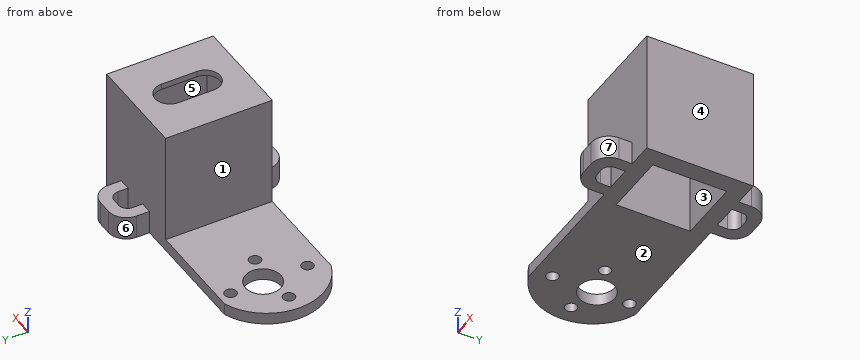
from build123d import *

# Parameters (mm, degrees)
SKETCH2_R            = 1
SKETCH2_R_2          = 3
BOSS_EXTRUDE2_DEPTH  = 2
SKETCH3_W            = 10.8
SKETCH3_H            = 12.5
CUT_EXTRUDE1_DEPTH   = 3
SKETCH4_W            = 17.364181201
SKETCH4_H            = 18
BOSS_EXTRUDE3_DEPTH  = 19
SKETCH5_W            = 10.8
SKETCH5_H            = 12.5
CUT_EXTRUDE2_DEPTH   = 18
BOSS_EXTRUDE4_DEPTH  = 4
FILLET1_R            = 1.5
FILLET2_R            = 3
FILLET1_OF_MIRROR1_R = 1.5
FILLET2_OF_MIRROR1_R = 3
CUT_EXTRUDE3_DEPTH   = 10


with BuildPart() as part:
    # Sketch2 → Boss-Extrude2 (new body)
    with BuildSketch(Plane.XY):
        with BuildLine():
            Line((-18.735484911, 68.428926153), (15.992877491, 68.428926153))
            Line((15.992877491, 68.428926153), (15.992877491, 50.428926153))
            Line((15.992877491, 50.428926153), (-18.735484911, 50.428926153))
            ThreePointArc((-18.735484911, 50.428926153), (-25.000050177, 59.428926153), (-18.735484911, 68.428926153))
        make_face()
        with Locations((-17, 53.428926153)):
            Circle(SKETCH2_R, mode=Mode.SUBTRACT)
        with Locations((-17, 60.928926153)):
            Circle(SKETCH2_R_2, mode=Mode.SUBTRACT)
        with Locations((-22, 59.428926153)):
            Circle(SKETCH2_R, mode=Mode.SUBTRACT)
        with Locations((-17, 66.428926153)):
            Circle(SKETCH2_R, mode=Mode.SUBTRACT)
        with Locations((-12, 59.428926153)):
            Circle(SKETCH2_R, mode=Mode.SUBTRACT)
    extrude(amount=BOSS_EXTRUDE2_DEPTH)

    # Sketch3 → Cut-Extrude1 (cut, through all)
    with BuildSketch(Plane.XY.offset(2)):
        with Locations((7.592877491, 59.428926153)):
            Rectangle(SKETCH3_W, SKETCH3_H)
    extrude(amount=-CUT_EXTRUDE1_DEPTH, mode=Mode.SUBTRACT)

    # Sketch4 → Boss-Extrude3 (add)
    with BuildSketch(Plane.XY.offset(2)):
        with Locations((7.310786891, 59.428926153)):
            Rectangle(SKETCH4_W, SKETCH4_H)
    extrude(amount=BOSS_EXTRUDE3_DEPTH)

    # Sketch5 → Cut-Extrude2 (cut)
    with BuildSketch(Plane(origin=(0, 0, 2), x_dir=(-1, 0, 0), z_dir=(0, 0, -1))):
        with Locations((-7.592877491, 59.428926153)):
            Rectangle(SKETCH5_W, SKETCH5_H)
    extrude(amount=-CUT_EXTRUDE2_DEPTH, mode=Mode.SUBTRACT)

    # Sketch7 → Boss-Extrude4 (add)
    with BuildSketch(Plane(origin=(0, 0, 0), x_dir=(-1, 0, 0), z_dir=(0, 0, -1))):
        Polygon((-11.692877491, 68.428926153), (-9.692877491, 68.428926153), (-9.692877491, 71.628926153), (-5.392877491, 71.628926153), (-5.392877491, 68.428926153), (-3.392877491, 68.428926153), (-3.392877491, 73.628926153), (-11.692877491, 73.628926153), align=None)
    boss_extrude4 = extrude(amount=-BOSS_EXTRUDE4_DEPTH)

    # Fillet1
    fillet1_edges = [part.edges().sort_by_distance(p)[0] for p in [
        (5.392877491, 71.628926153, 2),
        (9.692877491, 71.628926153, 2),
    ]]
    fillet(fillet1_edges, radius=FILLET1_R)

    # Fillet2
    fillet2_edges = [part.edges().sort_by_distance(p)[0] for p in [
        (3.392877491, 73.628926153, 2),
        (11.692877491, 73.628926153, 2),
    ]]
    fillet(fillet2_edges, radius=FILLET2_R)

    # Mirror1: Boss-Extrude4 across plane
    add(boss_extrude4.mirror(Plane.ZX.offset(59.428926153)))

    # Fillet1 of Mirror1
    fillet1_of_mirror1_edges = [part.edges().sort_by_distance(p)[0] for p in [
        (5.392877491, 47.228926153, 2),
        (9.692877491, 47.228926153, 2),
    ]]
    fillet(fillet1_of_mirror1_edges, radius=FILLET1_OF_MIRROR1_R)

    # Fillet2 of Mirror1
    fillet2_of_mirror1_edges = [part.edges().sort_by_distance(p)[0] for p in [
        (3.392877491, 45.228926153, 2),
        (11.692877491, 45.228926153, 2),
    ]]
    fillet(fillet2_of_mirror1_edges, radius=FILLET2_OF_MIRROR1_R)

    # Sketch9 → Cut-Extrude3 (cut)
    with BuildSketch(Plane.XY.offset(21)):
        with BuildLine():
            Line((9.971454774, 62.64486165), (9.971454774, 56.64486165))
            ThreePointArc((9.971454774, 56.64486165), (7.471454774, 54.14486165), (4.971454774, 56.64486165))
            Line((4.971454774, 56.64486165), (4.971454774, 62.64486165))
            ThreePointArc((4.971454774, 62.64486165), (7.471454774, 65.14486165), (9.971454774, 62.64486165))
        make_face()
    extrude(amount=-CUT_EXTRUDE3_DEPTH, mode=Mode.SUBTRACT)


solid = part.part
Input: part model. Units: mm. Frame: model coordinates. Face numbers are marked on the shaded views. A direction names the side the tool comes from. Give positions to 0.01 mm unless a question says otherwise; leave off trailing zeros. Write each loop counter-clockwise with the first axis right and the second up, starting at its lowest first coordinate (ties: lowest second). Pieces come first, ordered by that corner, then holes.
Q1. Section C-C, the plane x = -12. Output: boundary loops of the cut face in (y, z), plus the area to 3 significant figures.
Q2. Pull-direction query (Y, two-part tool) for the marked faces 4, 5, 6 and 7; classes: pulls with the +Y half, pulls with the -Y half, needs draft (parallel to the pull), parting line crosses it, or undercut.
Q3. First-contact query: P1, Ø4, axis at y = 68.5, z = 7.5, coming from the -X side; P2, Ø0.5, axis at y = 69, z = 1.5, coming from the -X side; P3, Ø2.5, axis at y = 49, z = 1.5, coming from the +X side; P4, Ø5, axis at x = -17, y = 60.93, coming from the -Z side. Flat tips, straight axial feed; report the tip coordinate or a pass-through.
Q4. Material intervals for probe 1 along Y at (x, z) = (-17, 0.7); probe 2 along X at (y, z) = (53.75, 16.5); probe 3 along X at (y, z) = (52.75, 19.25), sorted ascending.
Q5. Section A-A, the plane x = -17. Output: boundary loops of the cut face in (y, z), plus the area to 3 significant figures.
Q6. Set-up query: the marked faces 1, 2 and 3. Return all of +Z, -Z, +X, -X, +Y, -Y with unobstructed straight access to the full face (end or side cutting, diameter ignored); none if empty.
Q7. Section B-B, the plane z = 11.75. Output: boundary loops of the cut face in (x, y).
Q8. Section D-D, the plane y = 55. Output: boundary loops of the cut face in (x, z).
Filled in:
1. outline: (50.43, 0) - (58.43, 0) - (58.43, 2) - (50.43, 2) - close; (60.43, 0) - (68.43, 0) - (68.43, 2) - (60.43, 2) - close
1. area: 32.0 mm2
2. face 4: needs draft
2. face 5: undercut
2. face 6: pulls with the +Y half
2. face 7: pulls with the -Y half
3. P1: stops at x = -1.37
3. P2: stops at x = 3.39
3. P3: stops at x = 11.69
3. P4: passes through
4. probe 1: y = 50.43 to 52.43, 54.43 to 57.93, 63.93 to 65.43, 67.43 to 68.43
4. probe 2: x = -1.37 to 2.19, 12.99 to 15.99
4. probe 3: x = -1.37 to 15.99
5. outline: (50.43, 0) - (52.43, 0) - (52.43, 2) - (50.43, 2) - close; (54.43, 0) - (57.93, 0) - (57.93, 2) - (54.43, 2) - close; (63.93, 0) - (65.43, 0) - (65.43, 2) - (63.93, 2) - close; (67.43, 0) - (68.43, 0) - (68.43, 2) - (67.43, 2) - close
5. area: 16.0 mm2
6. face 1: +Z, -X, +Y, -Y
6. face 2: -Z, +X, -X, +Y, -Y
6. face 3: -Z
7. outline: (-1.37, 50.43) - (15.99, 50.43) - (15.99, 68.43) - (-1.37, 68.43) - close; hole (2.19, 53.18) - (12.99, 53.18) - (12.99, 65.68) - (2.19, 65.68) - close
8. outline: (-23.92, 0) - (2.19, 0) - (2.19, 20) - (5.59, 20) - (5.59, 21) - (-1.37, 21) - (-1.37, 2) - (-23.92, 2) - close; (9.35, 20) - (12.99, 20) - (12.99, 0) - (15.99, 0) - (15.99, 21) - (9.35, 21) - close
